Read the model definition and answer for the solid it produces. Units are mm, in the model's axes. Face numbers are marked on the shaded views. A direction names the side the tool comes from. Coordinates: 2 decimals unless noted, no trailing zeros. Write each loop counter-clockwise with the first axis right and the second up, starting at its lowest first coordinate (ties: lowest second). Pieces come first, ordered by that corner, then holes. Notation, with made-up numbers: (-11.75, 33.25) -> (21.25, 33.25) arc R6 cw to (21.25, 43.25) -> close; hole circle Ø2 at (69.5, -27). An arc over 180 degrees is marked (long way). Return JSON: item names as keys, results as strings.
from build123d import *

# Parameters (mm, degrees)
POCKET_DEPTH = 2


with BuildPart() as part:
    # Sketch → Revolution (revolve)
    with BuildSketch(Plane.YZ):
        Polygon((0, 0), (0, 2.385), (0.35507, 3), (7.75, 3), (10, 0.75), (10, 0), align=None)
    revolve(axis=Axis((0, 0, 0), (0, 1, 0)))

    # Sketch001 → Pocket (cut)
    with BuildSketch(Plane(origin=(0, 0, 0), x_dir=(0, 0, -1), z_dir=(0, -1, 0))):
        Polygon((-0.866025, -1.5), (0.866025, -1.5), (1.732051, 0), (0.866025, 1.5), (-0.866025, 1.5), (-1.732051, 0), align=None)
    extrude(amount=-POCKET_DEPTH, mode=Mode.SUBTRACT)


solid = part.part
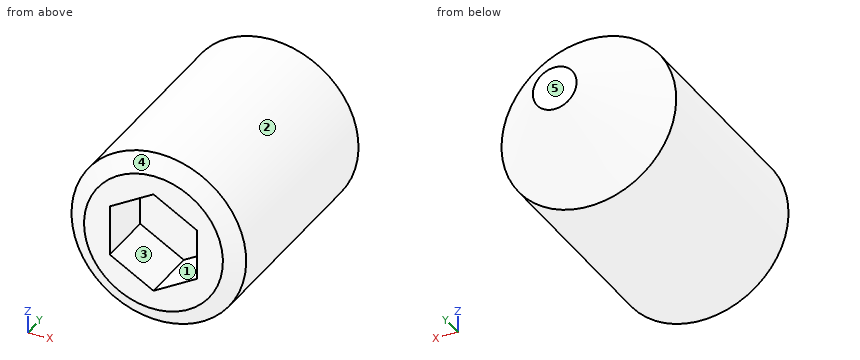
1. Consider L1, parallel to Z at x = 2.45, y = 1; L2, parallel to Z at x = 2.6, y = 5.75; L3, parallel to Y at x = 1.2, z = 1. Determine where each line is inside the solid, lowest interval first.
Taken from the geometry:
{"L1": "z = -1.73 to 1.73", "L2": "z = -1.5 to 1.5", "L3": "y = 2 to 9.19"}
2. The part is cut by section A-A (z = 0). Determine the outline of the cut face in (x, y) (3 decimals), then the cut area to 3 significant figures.
Taken from the geometry:
{"outline": "(-3, 0.355) -> (-2.385, 0) -> (-1.5, 0) -> (-1.5, 2) -> (1.5, 2) -> (1.5, 0) -> (2.385, 0) -> (3, 0.355) -> (3, 7.75) -> (0.75, 10) -> (-0.75, 10) -> (-3, 7.75) -> close", "area": "48.7 mm2"}
3. The part is cut by section B-B (y = 3.5). Determine the outline of the cut face in (x, z).
Taken from the geometry:
{"outline": "circle Ø6 at (0, 0)"}
4. A tool of negligible diameter and unlimited length cuts with its end or side. For the marked faces 1 and 2, from which of +Z, -Z, +X, -X, +Y, -Y can it reach the whole face along a straight path? Write none if from no direction.
Taken from the geometry:
{"face 1": "-Y", "face 2": "+Y, -Y"}
5. For a pull along X with two mould halves and no side action, classify the marked faces 3, 4 and 5 as +X half, -X half, draft (parallel to the pull), parting line (faces both ways), or undercut.
Taken from the geometry:
{"face 3": "undercut", "face 4": "parting line", "face 5": "draft"}
6. Flat-ended cylindrical pins translate along their axes: pin 1 Ø1.5 at (x, y) = (-1.5, 5) entering from +Z; pin 2 Ø0.5 at (y, z) = (1.5, -0.5) entering from -X; pin 3 Ø1 at (x, z) = (1, 2) entering from +Y. Find the tip coordinate at first contact, or state that the pin passes through.
Taken from the geometry:
{"pin 1": "stops at z = 2.9", "pin 2": "stops at x = -2.99", "pin 3": "stops at y = 9.01"}
